from build123d import *

# Parameters (mm, degrees)
BOSS_EXTRUDE1_DEPTH = 15
CUT_EXTRUDE1_REACH  = 57.908
SKETCH2_R           = 1.25
FILLET1_R           = 3
FILLET2_R           = 1


with BuildPart() as part:
    # Sketch1 → Boss-Extrude1 (new body)
    with BuildSketch(Plane.XY):
        Polygon((-21.874229857, 0), (-8.874229857, 0), (-8.874229857, 8.25), (40.125770143, 8.25), (40.125770143, 0), (53.125770143, 0), (53.125770143, 1.2), (41.925770143, 1.2), (41.925770143, 10.05), (-10.674229857, 10.05), (-10.674229857, 1.2), (-21.874229857, 1.2), align=None)
    extrude(amount=BOSS_EXTRUDE1_DEPTH)

    # Sketch2 → Cut-Extrude1 (cut, up to next)
    with BuildSketch(Plane(origin=(0, 1.2, 0), x_dir=(1, 0, 0), z_dir=(0, 1, 0)), mode=Mode.PRIVATE) as cut_extrude1_sk1:
        with Locations(Location((-18.374229857, -7.5, 0), (0, 0, 180))):
            Circle(SKETCH2_R)
    cut_extrude1_tool1 = extrude(cut_extrude1_sk1.sketch, amount=-CUT_EXTRUDE1_REACH, mode=Mode.PRIVATE) & part.part
    # Sketch2 → Cut-Extrude1 (cut, up to next)
    with BuildSketch(Plane(origin=(0, 1.2, 0), x_dir=(1, 0, 0), z_dir=(0, 1, 0)), mode=Mode.PRIVATE) as cut_extrude1_sk2:
        with Locations(Location((49.625770143, -7.5, 0), (0, 0, 180))):
            Circle(SKETCH2_R)
    cut_extrude1_tool2 = extrude(cut_extrude1_sk2.sketch, amount=-CUT_EXTRUDE1_REACH, mode=Mode.PRIVATE) & part.part
    add(cut_extrude1_tool1.solids().sort_by_distance((-18.37423, 1.2, 7.5))[0], mode=Mode.SUBTRACT)
    add(cut_extrude1_tool2.solids().sort_by_distance((49.62577, 1.2, 7.5))[0], mode=Mode.SUBTRACT)

    # Fillet1
    fillet1_edges = [part.edges().sort_by_distance(p)[0] for p in [
        (53.125770143, 0.6, 0),
        (-21.874229857, 0.6, 0),
        (-10.674229857, 1.2, 7.5),
        (41.925770143, 1.2, 7.5),
        (53.125770143, 0.6, 15),
        (-21.874229857, 0.6, 15),
    ]]
    fillet(fillet1_edges, radius=FILLET1_R)

    # Fillet2
    fillet2_edges = [part.edges().sort_by_distance(p)[0] for p in [
        (-10.674229857, 10.05, 7.5),
        (41.925770143, 10.05, 7.5),
    ]]
    fillet(fillet2_edges, radius=FILLET2_R)


solid = part.part
Design review of the part built by this model. Coordinates are the model's own, in mm. A direction names the side the tool comes from. Round coordinates to 2 decimals unless told otherwise and drop trailing zeros. Loops run counter-clockwise (first coordinate to the right, second up) from the corner with the lowest first, then second, coordinate; pieces in that order, holes last. Notation, with made-up numbers: M 59,14.5 L 96,14.5 A24 cw 96,26.5 Z; hole C 9.5,45 d7. An arc over 180 degrees is marked long. Answer as a JSON object with one key per item and string values.
Item 1: We need section B-B on y = 7.5. Give the boundary of the cut face in (x, z).
Answer sheet:
{"outline": "M -10.67,0 L -8.87,0 L -8.87,15 L -10.67,15 Z; M 40.13,0 L 41.93,0 L 41.93,15 L 40.13,15 Z"}
Item 2: Wall thickness on L1, parallel to X at y = 4, z = 5.5; L2, parallel to X at y = 9, z = 5; L3, parallel to Y at x = -6, z = 8.75: over which ranges is each line inside the solid? List them lowest first. Write a range as from..to.
Answer sheet:
{"L1": "x = -10.68..-8.87, 40.13..41.93", "L2": "x = -10.67..41.93", "L3": "y = 8.25..10.05"}
Item 3: We need section D-D on x = 9.5. Give the boundary of the cut face in (y, z).
Answer sheet:
{"outline": "M 8.25,0 L 10.05,0 L 10.05,15 L 8.25,15 Z"}
Item 4: We need section A-A on z = 7.5. Give the boundary of the cut face in (x, y), and give its area (3 significant figures).
Answer sheet:
{"outline": "M -21.87,0 L -19.62,0 L -19.62,1.2 L -21.87,1.2 Z; M -17.12,0 L -8.87,0 L -8.87,8.25 L 40.13,8.25 L 40.13,0 L 48.38,0 L 48.38,1.2 L 44.93,1.2 A3 cw 41.93,4.2 L 41.93,9.05 A1 ccw 40.93,10.05 L -9.67,10.05 A1 ccw -10.67,9.05 L -10.67,4.2 A3 cw -13.67,1.2 L -17.12,1.2 Z; M 50.88,0 L 53.13,0 L 53.13,1.2 L 50.88,1.2 Z", "area": "149 mm^2"}
Item 5: Clearance check with flat-ended pins moving along their axes: P1, Ø4, axis at y = 6.5, z = 4, coming from the -X side; P2, Ø1.5, axis at x = 4.5, z = 8.5, coming from the -Y side; P3, Ø4, axis at x = -19.5, z = 7, coming from the +Y side. State where each tip first meets the part, or that it passes through.
Answer sheet:
{"P1": "stops at x = -10.67", "P2": "stops at y = 8.25", "P3": "stops at y = 1.2"}
Item 6: Machinability: for faces 5 (the flat face through (40.126, 4, 7)), 6 (the flat face through (-17, 1.2, 7)), 7 (the flat face through (48, 1.2, 7)), which of the approach directions +Z, -Z, +X, -X, +Y, -Y give a long, thin tool a straight path to every point of the face, cutting with its end or side? Answer none if there is none.
Answer sheet:
{"face 5": "+Z, -Z, -Y", "face 6": "+Z, -Z, -X, +Y", "face 7": "+Z, -Z, +X, +Y"}
Item 7: The part is to be moulded in two halves that separate along Z. For faces 1 (the flat face through (15, 9, 0)), 2 (the cylindrical face through (49.05, 0.61, 6.39)), 3 (the cylindrical face through (-19.53, 0.61, 7.02)), 4 (the cylindrical face through (-11.576, 2.055, 7.605)), say which applies: pulls with the +Z half, pulls with the -Z half, needs draft (parallel to the pull), parting line crosses it, or undercut.
Answer sheet:
{"face 1": "pulls with the -Z half", "face 2": "undercut", "face 3": "undercut", "face 4": "needs draft"}
Item 8: We need section C-C on z = 10.5. Give the boundary of the cut face in (x, y), and give its area (3 significant figures).
Answer sheet:
{"outline": "M -21.87,0 L -8.87,0 L -8.87,8.25 L 40.13,8.25 L 40.13,0 L 53.13,0 L 53.13,1.2 L 44.93,1.2 A3 cw 41.93,4.2 L 41.93,9.05 A1 ccw 40.93,10.05 L -9.67,10.05 A1 ccw -10.67,9.05 L -10.67,4.2 A3 cw -13.67,1.2 L -21.87,1.2 Z", "area": "155 mm^2"}
